from build123d import *

# Parameters (mm, degrees)
ESQUISSE1_W             = 45
ESQUISSE1_H             = 32
BOSS_EXTRU_1_DEPTH      = 7.8
ESQUISSE2_W             = 41
ESQUISSE2_H             = 28
ENL_V_MAT_EXTRU_1_DEPTH = 7.5
ESQUISSE4_OUTSIDE_W     = 58.154
ESQUISSE4_OUTSIDE_H     = 45.154
ESQUISSE4_OUTSIDE_W_2   = 43
ESQUISSE4_OUTSIDE_H_2   = 30
ENL_V_MAT_EXTRU_2_DEPTH = 5
ESQUISSE5_W             = 9
ESQUISSE5_H             = 9
ENL_V_MAT_EXTRU_3_DEPTH = 5
ESQUISSE6_W             = 5
ESQUISSE6_H             = 5
BOSS_EXTRU_2_DEPTH      = 2.8


with BuildPart() as part:
    # Esquisse1 → Boss.-Extru.1 (new body)
    with BuildSketch(Plane.XY):
        with Locations((7.42437914, -4.08326268)):
            Rectangle(ESQUISSE1_W, ESQUISSE1_H)
    extrude(amount=BOSS_EXTRU_1_DEPTH)

    # Esquisse2 → Enlèv. mat.-Extru.1 (cut)
    with BuildSketch(Plane.XY.offset(7.8)):
        with Locations((7.42437914, -4.08326268)):
            Rectangle(ESQUISSE2_W, ESQUISSE2_H)
    extrude(amount=-ENL_V_MAT_EXTRU_1_DEPTH, mode=Mode.SUBTRACT)

    # Esquisse4 outside → Enlèv. mat.-Extru.2 (cut)
    with BuildSketch(Plane.XY.offset(7.8)):
        with Locations((7.424, -4.083)):
            Rectangle(ESQUISSE4_OUTSIDE_W, ESQUISSE4_OUTSIDE_H)
        with Locations((7.42437914, -4.08326268)):
            Rectangle(ESQUISSE4_OUTSIDE_W_2, ESQUISSE4_OUTSIDE_H_2, mode=Mode.SUBTRACT)
    extrude(amount=-ENL_V_MAT_EXTRU_2_DEPTH, mode=Mode.SUBTRACT)

    # Esquisse5 → Enlèv. mat.-Extru.3 (cut)
    with BuildSketch(Plane(origin=(0, 0, 0), x_dir=(-1, 0, 0), z_dir=(0, 0, -1))):
        with Locations((-19.42437914, -3.58326268)):
            Rectangle(ESQUISSE5_W, ESQUISSE5_H)
    extrude(amount=-ENL_V_MAT_EXTRU_3_DEPTH, mode=Mode.SUBTRACT)

    # Esquisse6 → Boss.-Extru.2 (add)
    with BuildSketch(Plane(origin=(0, 0, 0), x_dir=(-1, 0, 0), z_dir=(0, 0, -1))):
        with Locations((-27.42437914, -22.58326268)):
            Rectangle(ESQUISSE6_W, ESQUISSE6_H)
    extrude(amount=-BOSS_EXTRU_2_DEPTH)

    # Esquisse7 → Chambrage pour vis à tête ronde bombée M1.61 (revolve, cut)
    with BuildSketch(Plane(origin=(27.324958559, -22.78326268, 0), x_dir=(0, 1, 0), z_dir=(1, 0, 0))):
        Polygon((0, 0), (0, 7.790774557), (0.9, 7.25), (0.9, 1.3), (1.75, 1.3), (1.75, 0.025), (1.775, 0), align=None)
    revolve(axis=Axis((27.324958559, -22.78326268, -6.35), (0, 0, 1)), mode=Mode.SUBTRACT)


solid = part.part
Read the model definition and answer for the solid it produces. Units are mm, in the model's axes. A direction names the side the tool comes from. Give positions to 0.01 mm unless a question says otherwise; leave off trailing zeros. Write each loop counter-clockwise with the first axis right and the second up, starting at its lowest first coordinate (ties: lowest second). Pieces come first, ordered by that corner, then holes. Notation, with made-up numbers: M 87.5,23.5 L 106.5,23.5 A34 cw 106.5,54.5 Z; hole C 23,20.25 d7. An arc over 180 degrees is marked long. One line per item, written item: value. Start each with the question number.
(1) Find section A-A (y = -3). Determine the outline of the cut face in (x, z).
(2) Find section C-C (z = 2). Determine the outline of the cut face in (x, y).
(3) Flat-ended cylindrical pins translate along their axes: pin 1 Ø1.5 at (x, z) = (-6, 6.5) entering from +Y; pin 2 Ø2 at (x, y) = (10.5, -3) entering from +Z; pin 3 Ø2 at (x, y) = (27.32, -22.78) entering from -Z. Find the tip coordinate at first contact, or state that the pin passes through.
(4) Determine the mould class of faces 1 (the flat face through (7, 10.917, 5)), 2 (the flat face through (5, -20.083, 1)), 3 (the flat face through (27.924, -4, 4)) for opening direction Y: pulls with the +Y half, pulls with the -Y half, needs draft (parallel to the pull), parting line crosses it, or undercut.
(5) A tool of negligible diameter and unlimited length cuts with its end or side. For faces 4 (the flat face through (28, -24, 1.3)), 5 (the flat face through (28.924, -4, 5)), 6 (the flat face through (24.924, -23, 1)), from which of +Z, -Z, +X, -X, +Y, -Y can it reach the whole face along a straight path? Write none if from no direction.
(6) Find section B-B (x = 18). Determine the outline of the cut face in (y, z), plus the area to 3 significant figures.
(7) Find the intervals of material crossed by line 1 (X direction, y = 8.5, z = 4.5); line 2 (Y direction, x = -3.5, z = 4.25); line 3 (Y direction, x = -3, z = 1.5), in increasing order.
(8) Find section D-D (y = -16.5). Determine the outline of the cut face in (x, z).
Results below:
1. outline: M -15.08,0 L 14.92,0 L 14.92,0.3 L -13.08,0.3 L -13.08,7.8 L -14.08,7.8 L -14.08,2.8 L -15.08,2.8 Z; M 23.92,0 L 29.92,0 L 29.92,2.8 L 28.92,2.8 L 28.92,7.8 L 27.92,7.8 L 27.92,0.3 L 23.92,0.3 Z
2. outline: M -15.08,-20.08 L 24.92,-20.08 L 24.92,-25.08 L 29.92,-25.08 L 29.92,11.92 L -15.08,11.92 Z; hole M -13.08,-18.08 L 27.92,-18.08 L 27.92,9.92 L -13.08,9.92 Z; hole C 27.32,-22.78 d1.8
3. pin 1: stops at y = 10.92
3. pin 2: stops at z = 0.3
3. pin 3: stops at z = 1.3
4. face 1: pulls with the +Y half
4. face 2: pulls with the -Y half
4. face 3: undercut
5. face 4: -Z
5. face 5: +Z, +X, +Y, -Y
5. face 6: +Z, -Z, -X, -Y
6. outline: M -20.08,0 L -8.08,0 L -8.08,0.3 L -18.08,0.3 L -18.08,7.8 L -19.08,7.8 L -19.08,2.8 L -20.08,2.8 Z; M 0.92,0 L 11.92,0 L 11.92,2.8 L 10.92,2.8 L 10.92,7.8 L 9.92,7.8 L 9.92,0.3 L 0.92,0.3 Z
6. area: 26.9 mm^2
7. line 1: x = -14.08 to -13.08, 27.92 to 28.92
7. line 2: y = -19.08 to -18.08, 9.92 to 10.92
7. line 3: y = -20.08 to -18.08, 9.92 to 11.92
8. outline: M -15.08,0 L 29.92,0 L 29.92,2.8 L 28.92,2.8 L 28.92,7.8 L 27.92,7.8 L 27.92,0.3 L -13.08,0.3 L -13.08,7.8 L -14.08,7.8 L -14.08,2.8 L -15.08,2.8 Z
